from build123d import *

# Parameters (mm, degrees)
F0_R     = 36.6966973779
F1_DEPTH = 50.8
F2_R     = 5.08
F3_R     = 23.8679289638
F4_DEPTH = 13.208
F5_DEPTH = 25.4
F6_R     = 5.08
F7_SIZE  = 5.08
F8_R     = 2.54


# Not quite as in the source:
# - two fillets or chamfers of one size are made in one step


with BuildPart() as f1:
    # F0 (on Top) → F1 (new body)
    with BuildSketch(Plane.XY):
        Circle(F0_R)
    extrude(amount=F1_DEPTH)

    # F2
    f2_edges = [f1.edges().sort_by_distance(p)[0] for p in [
        (-36.696697, 0, 50.8),
    ]]
    fillet(f2_edges, radius=F2_R)

    # F3 (on face) → F4 (cut)
    with BuildSketch(Plane.XY.offset(50.8)):
        Circle(F3_R)
    extrude(amount=-F4_DEPTH, mode=Mode.SUBTRACT)

    # F5 (add): a face of the model
    f5_faces = [f1.faces().sort_by_distance(p)[0] for p in [
        (-30.7224421333, 0, 50.8),
    ]]
    extrude(f5_faces, amount=F5_DEPTH)

    # F6
    f6_edges = [f1.edges().sort_by_distance(p)[0] for p in [
        (-31.616697, 0, 50.8),
    ]]
    fillet(f6_edges, radius=F6_R)

    # F7
    f7_edges = [f1.edges().sort_by_distance(p)[0] for p in [
        (-31.616697, 0, 76.2),
    ]]
    chamfer(f7_edges, length=F7_SIZE)

    # F8
    f8_edges = [f1.edges().sort_by_distance(p)[0] for p in [
        (-31.616697, 0, 71.12),
        (-26.536697, 0, 76.2),
    ]]
    fillet(f8_edges, radius=F8_R)


solid = f1.part
Design review of the part built by this model. Coordinates are the model's own, in mm. A direction names the side the tool comes from. Give positions to 0.01 mm unless a question says otherwise; leave off trailing zeros. Loops run counter-clockwise (first coordinate to the right, second up) from the corner with the lowest first, then second, coordinate; pieces in that order, holes last. Notation, with made-up numbers: M 72.5,82.25 L 120.5,82.25 A25 ccw 120.5,115.25 Z; hole C 37.5,-34.75 d8. An arc over 180 degrees is marked long. Write item = value, one per line.
Q1. For faces 1 (the flat face through (-1, 1, 0)), 2 (the cylindrical face through (-5.17, -23.3, 56.63)), list the 3-axis set-ups (+Z, -Z, +X, -X, +Y, -Y) from which the entire face can be reached by the end or side of a thin tool; tool diameter is ignored.
Output values:
face_1 = -Z, +X, -X, +Y, -Y
face_2 = +Z
Q2. We need section B-B (z = 11). Give the boundary of the cut face in (x, y), plus the area to 3 significant figures.
Output values:
outline = C 0,0 d73.39
area = 4,230 mm^2
Q3. Insertion check: pin 1 (12 mm diameter, centred on y = -17, z = 11.5, fed in from -X); pin 2 (2 mm diameter, centred on x = 17, z = 60.5, fed in from -Y); pin 3 (10 mm diameter, centred on y = 21, z = 9, fed in from -X). Each pin has a flat end and moves straight along its axis. Give the tip position at first contact, or say it passes through.
Output values:
pin_1 = -35.01
pin_2 = -27.27
pin_3 = -33.02
Q4. We need section A-A (z = 39.5). Give the boundary of the cut face in (x, y).
Output values:
outline = C 0,0 d73.39; hole C 0,0 d47.74
Q5. To check wall thickness, follow line 1 (Y direction, x = 0, z = 57); line 2 (Z direction, x = -14, y = -14.5); line 3 (Y direction, x = 0, z = 14). State the ranges of each line that lie inside material, in increasing order. Write a range as [from, to].
Output values:
line_1 = [-31.62, -23.87], [23.87, 31.62]
line_2 = [0, 37.59]
line_3 = [-36.7, 36.7]
Q6. Draft analysis for pull direction X (two halves, no side actions). For faces 3 (the cylindrical face through (-7.955, -35.824, 22.54)), 4 (the flat face through (-23, -7, 76.2)), 5 (the flat face through (0, 0, 37.592)), state which applies: +X half, -X half, draft (parallel to the pull), parting line (faces both ways), or undercut.
Output values:
face_3 = parting line
face_4 = draft
face_5 = undercut
